from build123d import *

# Parameters (mm, degrees)
ESQUISSE1_W             = 70
ESQUISSE1_H             = 200
BOSS_EXTRU_1_DEPTH      = 5
BOSS_EXTRU_2_DEPTH      = 100
ESQUISSE3_W             = 70
ESQUISSE3_H             = 200
BOSS_EXTRU_3_DEPTH      = 5
ENL_V_MAT_EXTRU_2_DEPTH = 5
CONG_3_R                = 1
ESQUISSE7_R             = 1.75
ENL_V_MAT_EXTRU_4_DEPTH = 5
ENL_V_MAT_EXTRU_5_DEPTH = 2
ESQUISSE9_W             = 25
ESQUISSE9_H             = 25
ENL_V_MAT_EXTRU_6_DEPTH = 25
CONG_4_R                = 2


with BuildPart() as part:
    # Esquisse1 → Boss.-Extru.1 (new body)
    with BuildSketch(Plane.XY):
        with Locations((-35, 100)):
            Rectangle(ESQUISSE1_W, ESQUISSE1_H)
    extrude(amount=BOSS_EXTRU_1_DEPTH)

    # Esquisse2 → Boss.-Extru.2 (add)
    with BuildSketch(Plane.XY.offset(5)):
        Polygon((0, 0), (-70, 0), (-70, 5), (-5, 5), (-5, 195), (-70, 195), (-70, 200), (0, 200), align=None)
    extrude(amount=BOSS_EXTRU_2_DEPTH)

    # Esquisse3 → Boss.-Extru.3 (add)
    with BuildSketch(Plane.XY.offset(105)):
        with Locations((-35, 100)):
            Rectangle(ESQUISSE3_W, ESQUISSE3_H)
    extrude(amount=BOSS_EXTRU_3_DEPTH)

    # Esquisse5 → Enl_v. mat.-Extru.2 (cut)
    with BuildSketch(Plane.XZ):
        with BuildLine():
            ThreePointArc((-65.636494811, 17.582146985), (-67.179174329, 14.605555398), (-70, 12.793677891))
            Line((-70, 12.793677891), (-70, 7.3))
            ThreePointArc((-70, 7.3), (-69.707199718, 7.315923251), (-69.417853015, 7.363505189))
            ThreePointArc((-69.417853015, 7.363505189), (-63.569041252, 10.569041252), (-60.363505189, 16.417853015))
            ThreePointArc((-60.363505189, 16.417853015), (-62.417853015, 19.636494811), (-65.636494811, 17.582146985))
        make_face()
        with BuildLine():
            ThreePointArc((-60.363505189, 94.417853015), (-63.292800282, 92.315923251), (-65.7, 95))
            Line((-65.7, 95), (-65.7, 95.320415964))
            ThreePointArc((-65.7, 95.320415964), (-67.270907084, 92.506959978), (-70, 90.793677891))
            Line((-70, 90.793677891), (-70, 85.3))
            ThreePointArc((-70, 85.3), (-69.707199718, 85.315923251), (-69.417853015, 85.363505189))
            ThreePointArc((-69.417853015, 85.363505189), (-63.569041252, 88.569041252), (-60.363505189, 94.417853015))
        make_face()
        with BuildLine():
            Line((-65.7, 95.320415964), (-65.7, 95))
            ThreePointArc((-65.7, 95), (-63.292800282, 92.315923251), (-60.363505189, 94.417853015))
            ThreePointArc((-60.363505189, 94.417853015), (-60.315923251, 94.707199718), (-60.3, 95))
            ThreePointArc((-60.3, 95), (-62.707199718, 97.684076749), (-65.636494811, 95.582146985))
            ThreePointArc((-65.636494811, 95.582146985), (-65.666891669, 95.450952525), (-65.7, 95.320415964))
        make_face()
        with BuildLine():
            Line((-65.7, 100), (-65.7, 95.320415964))
            ThreePointArc((-65.7, 95.320415964), (-65.666891669, 95.450952525), (-65.636494811, 95.582146985))
            ThreePointArc((-65.636494811, 95.582146985), (-62.707199718, 97.684076749), (-60.3, 95))
            Line((-60.3, 95), (-60.3, 100))
            ThreePointArc((-60.3, 100), (-63, 102.7), (-65.7, 100))
        make_face()
    enl_v_mat_extru_2 = extrude(amount=-ENL_V_MAT_EXTRU_2_DEPTH, mode=Mode.SUBTRACT)

    # Sym_trie1: Enl_v. mat.-Extru.2 across plane
    add(enl_v_mat_extru_2.mirror(Plane.ZX.offset(100)), mode=Mode.SUBTRACT)

    # Cong_3
    # the kernel refuses this fillet: 1 mm, written as the material it takes off along each edge
    with BuildSketch(Plane(origin=(-70, 5, 10), x_dir=(-0.7991819531537966, 0, -0.6010891828616473), z_dir=(-0.6010891828616473, 0, 0.7991819531537966))) as cong_3_piece_1_section:
        with BuildLine():
            CenterArc((2.7 + CONG_3_R, CONG_3_R), CONG_3_R, 180, 90)
            Line((2.7 + CONG_3_R, 0), (2.7, 0))
            Line((2.7, 0), (2.7, CONG_3_R))
        make_face()
    cong_3_piece_1 = revolve(axis=Axis((-70, 5, 10), (0, -1, 0)), revolution_arc=65.503372271, mode=Mode.PRIVATE)
    cong_3_piece_1 = cong_3_piece_1 & Plane(origin=(-71.983611948, 4.575730045, 18.983611948), x_dir=(0.21560999438500908, 0, -0.9764795596023996), z_dir=(0, -1, 0)) * Cylinder(11.9, 15, mode=Mode.PRIVATE)
    add(cong_3_piece_1, mode=Mode.SUBTRACT)
    with BuildSketch(Plane(origin=(-70, -2.166523883, 7.3), x_dir=(0, 0, -1), z_dir=(0, 1, 0)), Plane(origin=(-70, -2.166523883, 85.3), x_dir=(0, 0, -1), z_dir=(0, 1, 0))) as cong_3_piece_2:
        with BuildLine():
            CenterArc((0.866609553, -1), CONG_3_R, 90, 76.627101296)
            Line((-0.106275834, -0.768712252), (-0.203564373, -0.745583477))
            ThreePointArc((-0.203564373, -0.745583477), (-0.161153145, -0.560585985), (-0.1, 0))
            Line((-0.1, 0), (0, 0.1))
            Line((0, 0.1), (0.866609553, 0.1))
            Line((0.866609553, 0.1), (0.866609553, 0))
        make_face()
    extrude(amount=9.333047767, mode=Mode.SUBTRACT)
    with BuildSketch(Plane(origin=(-70, -4.265669235, 12.793677891), x_dir=(0.904005218558232, 0, 0.4275214203048584), z_dir=(0, 1, 0)), Plane(origin=(-70, -4.265669235, 90.793677891), x_dir=(0.9040052185582337, 0, 0.42752142030485457), z_dir=(0, 1, 0))) as cong_3_piece_3:
        with BuildLine():
            CenterArc((1.575016333, -0.991349121), CONG_3_R, 82.458090337, 122.852275444)
            Line((0.671011114, -1.418870542), (0, 0))
            ThreePointArc((0, 0), (0.853133847, 0.056230712), (1.706267694, 0))
        make_face()
    extrude(amount=13.53133847, mode=Mode.SUBTRACT)
    with BuildSketch(Plane(origin=(-70, 0, 10), x_dir=(-0.7991819531537966, 0, -0.6010891828616473), z_dir=(-0.6010891828616473, 0, 0.7991819531537966))) as cong_3_piece_4_section:
        with BuildLine():
            CenterArc((2.7 + CONG_3_R, -CONG_3_R), CONG_3_R, 90, 90)
            Line((2.7, -CONG_3_R), (2.7, 0))
            Line((2.7, 0), (2.7 + CONG_3_R, 0))
        make_face()
    cong_3_piece_4 = revolve(axis=Axis((-70, 0, 10), (0, -1, 0)), revolution_arc=65.503372271, mode=Mode.PRIVATE)
    cong_3_piece_4 = cong_3_piece_4 & Plane(origin=(-71.983611948, 0.424269944, 18.983611948), x_dir=(0.21560999438500908, 0, -0.9764795596023996), z_dir=(0, -1, 0)) * Cylinder(11.9, 15, mode=Mode.PRIVATE)
    add(cong_3_piece_4, mode=Mode.SUBTRACT)
    with BuildSketch(Plane(origin=(-70, 5, 88), x_dir=(-0.7991819531536386, 0, -0.6010891828618574), z_dir=(-0.6010891828618574, 0, 0.7991819531536386))) as cong_3_piece_5_section:
        with BuildLine():
            CenterArc((2.7 + CONG_3_R, CONG_3_R), CONG_3_R, 180, 90)
            Line((2.7 + CONG_3_R, 0), (2.7, 0))
            Line((2.7, 0), (2.7, CONG_3_R))
        make_face()
    cong_3_piece_5 = revolve(axis=Axis((-70, 5, 88), (0, -1, 0)), revolution_arc=65.503372271, mode=Mode.PRIVATE)
    cong_3_piece_5 = cong_3_piece_5 & Plane(origin=(-71.983611948, 4.575730059, 96.983611948), x_dir=(0.2156099943850066, 0, -0.9764795596024002), z_dir=(0, -1, 0)) * Cylinder(11.9, 15, mode=Mode.PRIVATE)
    add(cong_3_piece_5, mode=Mode.SUBTRACT)
    with BuildSketch(Plane(origin=(-70, 0, 88), x_dir=(-0.7991819531536386, 0, -0.6010891828618574), z_dir=(-0.6010891828618574, 0, 0.7991819531536386))) as cong_3_piece_6_section:
        with BuildLine():
            CenterArc((2.7 + CONG_3_R, -CONG_3_R), CONG_3_R, 90, 90)
            Line((2.7, -CONG_3_R), (2.7, 0))
            Line((2.7, 0), (2.7 + CONG_3_R, 0))
        make_face()
    cong_3_piece_6 = revolve(axis=Axis((-70, 0, 88), (0, -1, 0)), revolution_arc=65.503372271, mode=Mode.PRIVATE)
    cong_3_piece_6 = cong_3_piece_6 & Plane(origin=(-71.983611948, 0.424269931, 96.983611948), x_dir=(0.2156099943850066, 0, -0.9764795596024002), z_dir=(0, -1, 0)) * Cylinder(11.9, 15, mode=Mode.PRIVATE)
    add(cong_3_piece_6, mode=Mode.SUBTRACT)

    # Esquisse7 → Enl_v. mat.-Extru.4 (cut)
    with BuildSketch(Plane.XY.offset(110)):
        with Locations((-55.5, 23)):
            Circle(ESQUISSE7_R)
        with Locations((-35.5, 23)):
            Circle(ESQUISSE7_R)
        with Locations(Location((-55.5, 177, 0), (0, 0, 180))):
            Circle(ESQUISSE7_R)
        with Locations(Location((-35.5, 177, 0), (0, 0, 180))):
            Circle(ESQUISSE7_R)
    extrude(amount=-ENL_V_MAT_EXTRU_4_DEPTH, mode=Mode.SUBTRACT)

    # Esquisse8 → Enl_v. mat.-Extru.5 (cut)
    with BuildSketch(Plane(origin=(0, 0, 105), x_dir=(-1, 0, 0), z_dir=(0, 0, -1))):
        Polygon((33.854551733, 25.85), (37.145448267, 25.85), (38.790896534, 23), (37.145448267, 20.15), (33.854551733, 20.15), (32.209103466, 23), align=None)
        Polygon((53.854551733, 25.85), (57.145448267, 25.85), (58.790896534, 23), (57.145448267, 20.15), (53.854551733, 20.15), (52.209103466, 23), align=None)
        Polygon((52.209103466, 177), (53.854551733, 174.15), (57.145448267, 174.15), (58.790896534, 177), (57.145448267, 179.85), (53.854551733, 179.85), align=None)
        Polygon((32.209103466, 177), (33.854551733, 174.15), (37.145448267, 174.15), (38.790896534, 177), (37.145448267, 179.85), (33.854551733, 179.85), align=None)
    extrude(amount=-ENL_V_MAT_EXTRU_5_DEPTH, mode=Mode.SUBTRACT)

    # Esquisse9 → Enl_v. mat.-Extru.6 (cut)
    with BuildSketch(Plane(origin=(0, 0, 0), x_dir=(-1, 0, 0), z_dir=(0, 0, -1))):
        with Locations((22.5, 187.5)):
            Rectangle(ESQUISSE9_W, ESQUISSE9_H)
    extrude(amount=-ENL_V_MAT_EXTRU_6_DEPTH, mode=Mode.SUBTRACT)

    # Cong_4
    cong_4_edges = [part.edges().sort_by_distance(p)[0] for p in [
        (-22.5, 195, 25),
        (-10, 195, 15),
        (-35, 195, 15),
        (-35, 200, 12.5),
        (-22.5, 175, 5),
        (-10, 185, 5),
        (-22.5, 200, 25),
        (-10, 200, 12.5),
        (-35, 185, 5),
        (-10, 187.5, 0),
        (-22.5, 175, 0),
        (-35, 187.5, 0),
    ]]
    fillet(cong_4_edges, radius=CONG_4_R)


solid = part.part
The model under review builds one solid part; all positions refer to its coordinate system, in mm. A direction names the side the tool comes from. Round coordinates to 2 decimals unless told otherwise and drop trailing zeros. Loops run counter-clockwise (first coordinate to the right, second up) from the corner with the lowest first, then second, coordinate; pieces in that order, holes last. Notation, with made-up numbers: (-8, 43.5) -> (39, 43.5) arc R11 cw to (39, 56.5) -> close; hole circle Ø3 at (61.25, -19). An arc over 180 degrees is marked (long way). Answer as CSV lines item,"result".
1) Add section A-A on z = 82. Write out the cut boundary in (x, y).
Geometry results:
outline,"(-70, 0) -> (0, 0) -> (0, 200) -> (-70, 200) -> (-70, 195) -> (-5, 195) -> (-5, 5) -> (-70, 5) -> close"
2) Add section B-B on x = -63. Write out the cut boundary in (y, z), plus the area to 3 significant figures.
Geometry results:
outline,"(0, 0) -> (200, 0) -> (200, 11.18) -> (195, 11.18) -> (195, 5) -> (5, 5) -> (5, 11.18) -> (0, 11.18) -> close; (0, 19.7) -> (5, 19.7) -> (5, 89.18) -> (0, 89.18) -> close; (0, 102.7) -> (5, 102.7) -> (5, 105) -> (195, 105) -> (195, 102.7) -> (200, 102.7) -> (200, 110) -> (0, 110) -> close; (195, 19.7) -> (200, 19.7) -> (200, 89.18) -> (195, 89.18) -> close"
area,"2,780 mm²"
3) Draft analysis for pull direction Y (two halves, no side actions). For faces 5 (the face through (-35, 0, 54)), 6 (the face through (-38, 101, 105)), 7 (the face through (-67.15, 197.54, 14.64)), state which applies: pulls with the +Y half, pulls with the -Y half, needs draft (parallel to the pull), parting line crosses it, or undercut.
Geometry results:
face 5,"pulls with the -Y half"
face 6,"undercut"
face 7,"needs draft"
4) Add section D-D on x = -29.5. Write out the cut boundary in (y, z), plus the area to 3 significant figures.
Geometry results:
outline,"(0, 0) -> (173, 0) arc R2 ccw to (175, 2) -> (175, 3) arc R2 ccw to (173, 5) -> (5, 5) -> (5, 105) -> (195, 105) -> (195, 27) arc R2 ccw to (197, 25) -> (198, 25) arc R2 ccw to (200, 27) -> (200, 110) -> (0, 110) -> close"
area,"2,770 mm²"
5) Tool access review of faces 1 (the face through (-38, 5, 54)), 2 (the face through (-63.64, 197.54, 88.5)), 3 (the face through (-34.1, 24.3, 107)), 4 (the face through (-10, 197.5, 8.3)): name each direction out of +Z, -Z, +X, -X, +Y, -Y from which nothing blocks a thin tool from reaching the whole face with its end or side.
Geometry results:
face 1,"-X"
face 2,"+Y, -Y"
face 3,"none"
face 4,"-Z, +Y"
6) To check wall thickness, follow line 1 along X through (y, z) = (177, 109); line 2 along Y through (x, z) = (-55.5, 108.25); line 3 along Z through (x, y) = (-63, 62). State the ranges of each line that lie inside material, in increasing order. Write a range as from..to.
Geometry results:
line 1,"x = -70..-57.25, -53.75..-37.25, -33.75..0"
line 2,"y = 0..21.25, 24.75..175.25, 178.75..200"
line 3,"z = 0..5, 105..110"
7) For P1, Ø10, axis at y = 101, z = 61.5, coming from the -X side, flat-tipped, find the tip position at first contact; note if it passes through.
Geometry results:
P1,"stops at x = -5"
8) Add section C-C on y = 132. Write out the cut boundary in (x, z).
Geometry results:
outline,"(-70, 0) -> (0, 0) -> (0, 110) -> (-70, 110) -> (-70, 105) -> (-5, 105) -> (-5, 5) -> (-70, 5) -> close"
